Part model, mm, in its own coordinate system. Face numbers are marked on the shaded views. A direction names the side the tool comes from. Coordinates: 2 decimals unless noted, no trailing zeros. Loops run counter-clockwise (first coordinate to the right, second up) from the corner with the lowest first, then second, coordinate; pieces in that order, holes last. Notation, with made-up numbers: (75, 6.25) - (98, 6.25) arc R22 ccw to (98, 27.25) - close; hole circle Ø1 at (45, 71). An arc over 180 degrees is marked (long way). Answer as CSV lines item,"result".
from build123d import *

# Parameters (mm, degrees)
SKETCH1_W                 = 42.1
SKETCH1_H                 = 42.1
BOSS_EXTRUDE1_DEPTH       = 8
CHAMFER1_SIZE             = 4
SKETCH2_R                 = 11
SKETCH2_R_2               = 5
BOSS_EXTRUDE2_DEPTH       = 2
CHAMFER2_SIZE             = 0.1
M2X0_4_TAPPED_HOLE1_D     = 1.6
M2X0_4_TAPPED_HOLE1_DEPTH = 8
M2X0_4_TAPPED_HOLE1_TIP   = 0.480688495


with BuildPart() as part:
    # Sketch1 → Boss-Extrude1 (new body)
    with BuildSketch(Plane(origin=(0, 0, 0), x_dir=(1, 0, 0), z_dir=(0, 1, 0))):
        Rectangle(SKETCH1_W, SKETCH1_H)
    extrude(amount=BOSS_EXTRUDE1_DEPTH)

    # Chamfer1
    chamfer1_edges = [part.edges().sort_by_distance(p)[0] for p in [
        (21.05, 4, 21.05),
        (-21.05, 4, 21.05),
        (-21.05, 4, -21.05),
        (21.05, 4, -21.05),
    ]]
    chamfer(chamfer1_edges, length=CHAMFER1_SIZE)

    # Sketch2 → Boss-Extrude2 (add)
    with BuildSketch(Plane(origin=(0, 8, 0), x_dir=(1, 0, 0), z_dir=(0, 1, 0))):
        Circle(SKETCH2_R)
        Circle(SKETCH2_R_2, mode=Mode.SUBTRACT)
    extrude(amount=BOSS_EXTRUDE2_DEPTH)

    # Chamfer2
    chamfer2_edges = [part.edges().sort_by_distance(p)[0] for p in [
        (-11, 8, 0),
        (-11, 10, 0),
    ]]
    chamfer(chamfer2_edges, length=CHAMFER2_SIZE)

    # M2x0.4 Tapped Hole1
    with Locations(Plane(origin=(-15.5, 8, -15.5), x_dir=(0, 0, 1), z_dir=(0, 1, 0))):
        with Locations((0, 0), (0, 31), (31, 31), (31, 0)):
            Hole(M2X0_4_TAPPED_HOLE1_D / 2, depth=M2X0_4_TAPPED_HOLE1_DEPTH)
            with Locations((0, 0, -(M2X0_4_TAPPED_HOLE1_DEPTH + M2X0_4_TAPPED_HOLE1_TIP / 2))):  # 118° drill point
                Cone(0, M2X0_4_TAPPED_HOLE1_D / 2, M2X0_4_TAPPED_HOLE1_TIP, mode=Mode.SUBTRACT)


solid = part.part
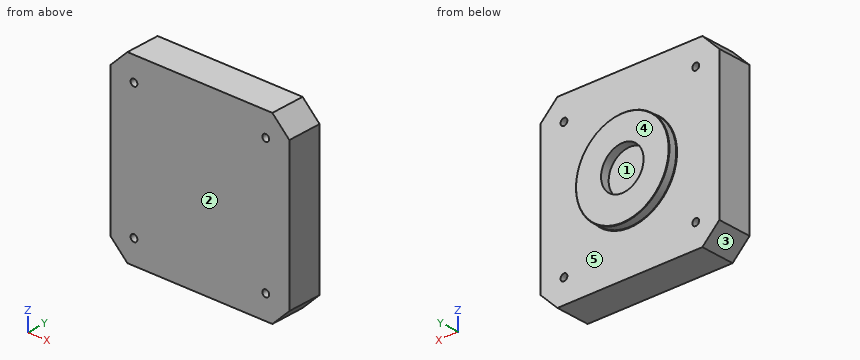
Q1. Two-plate mould, pull along Z, no slides. Class the marked faces 1, 2 and 3: released by +Z, released by -Z, zero draft, split by the parting line, or undercut.
Results:
face 1,"undercut"
face 2,"zero draft"
face 3,"released by -Z"
Q2. Saw through at B-B (x = 15.5). Give the cut face in (y, z), then the cut area to 3 significant figures.
Results:
outline,"(0, -21.05) - (8, -21.05) - (8, -16.3) - (0, -16.3) - close; (0, -14.7) - (8, -14.7) - (8, 14.7) - (0, 14.7) - close; (0, 16.3) - (8, 16.3) - (8, 21.05) - (0, 21.05) - close"
area,"311 mm^2"
Q3. Saw through at A-A (z = -15.5). Give the cut face in (x, y).
Results:
outline,"(-21.05, 0) - (-16.3, 0) - (-16.3, 8) - (-21.05, 8) - close; (-14.7, 0) - (14.7, 0) - (14.7, 8) - (-14.7, 8) - close; (16.3, 0) - (21.05, 0) - (21.05, 8) - (16.3, 8) - close"
Q4. Saw through at C-C (y = 5). Give the cut face in (x, z).
Results:
outline,"(-21.05, -17.05) - (-17.05, -21.05) - (17.05, -21.05) - (21.05, -17.05) - (21.05, 17.05) - (17.05, 21.05) - (-17.05, 21.05) - (-21.05, 17.05) - close; hole circle Ø1.6 at (-15.5, -15.5); hole circle Ø1.6 at (-15.5, 15.5); hole circle Ø1.6 at (15.5, -15.5); hole circle Ø1.6 at (15.5, 15.5)"
Q5. Which spindle directions (+Z, -Z, +X, -X, +Y, -Y) get a long thin tool onto all of the face, cutting with end or side? Do the marked faces 4 and 5. Say none if no direction does.
Results:
face 4,"+Z, -Z, +X, -X, +Y"
face 5,"+Y"
Q6. Wall check: L1, parallel to X at y = 3.5, z = -15.5; L2, parallel to Z at x = 0, y = 8.4. Give the ranges that are in metal, low to high.
Results:
L1,"x = -21.05 to -16.3, -14.7 to 14.7, 16.3 to 21.05"
L2,"z = -11 to -5, 5 to 11"
Q7. Saw through at D-D (z = 0). Give the cut face in (x, y).
Results:
outline,"(-21.05, 0) - (21.05, 0) - (21.05, 8) - (11.1, 8) - (11, 8.1) - (11, 9.9) - (10.9, 10) - (5, 10) - (5, 8) - (-5, 8) - (-5, 10) - (-10.9, 10) - (-11, 9.9) - (-11, 8.1) - (-11.1, 8) - (-21.05, 8) - close"
Q8. Flat gauge pin, fed straight in: pin 1 (1.8 mm diameter, centred on x = 15.5, z = 15.5, fed in from +Y). Where does the tip first touch, or does it go through?
Results:
pin 1,"stops at y = 8"
